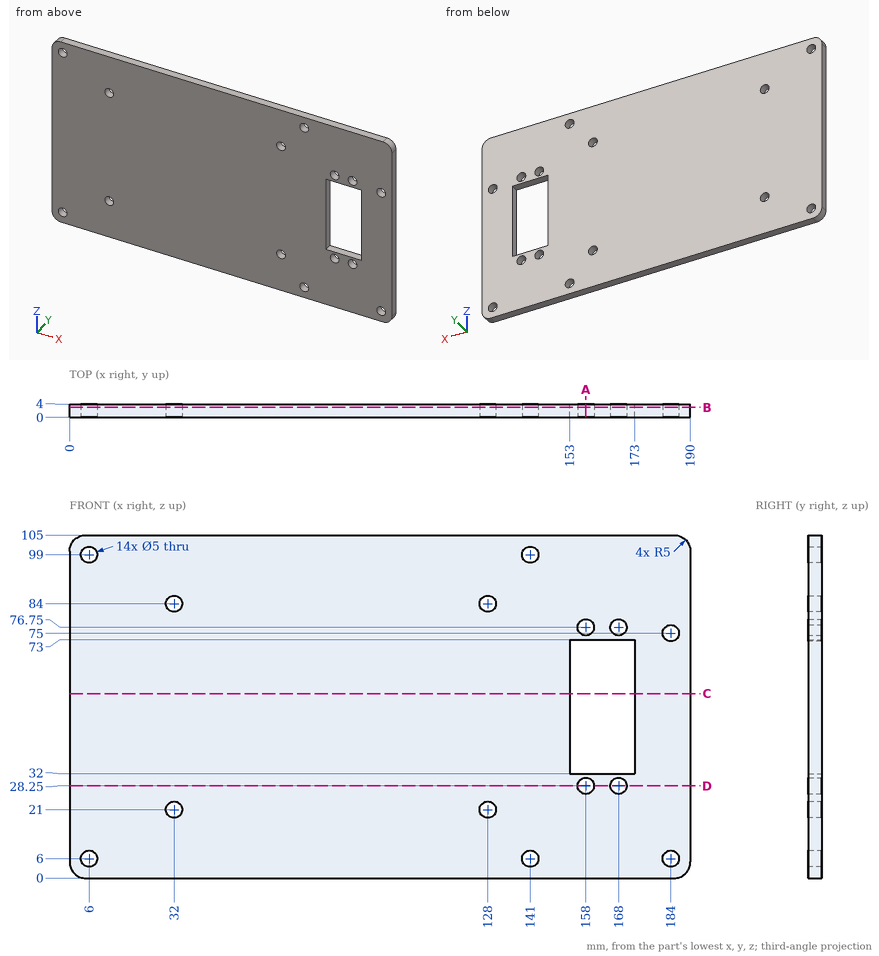
Design review of the part shown in the three views and the two pictorial views. Dimensions are in mm from the part's minimum x, y and z. Round coordinates to 2 decimals unless told otherwise and drop trailing zeros. Loops run counter-clockwise (first coordinate to the right, second up) from the corner with the lowest first, then second, coordinate; pieces in that order, holes last.
1) Wall thickness on line 1 along Z through (x, y) = (128, 3); line 2 along X through (y, z) = (2.55, 6); line 3 along X through (y, z) = (1.8, 84): over which ranges is each line inside the solid? List them lowest first.
Values follow:
line 1: z = 0 to 18.5, 23.5 to 81.5, 86.5 to 105
line 2: x = 0 to 3.5, 8.5 to 138.5, 143.5 to 181.5, 186.5 to 190
line 3: x = 0 to 29.5, 34.5 to 125.5, 130.5 to 190
2) Consider section D-D on z = 28.25. State the section outline as (x, y) points.
Values follow:
outline: (0, 0) - (155.5, 0) - (155.5, 4) - (0, 4) - close; (160.5, 0) - (165.5, 0) - (165.5, 4) - (160.5, 4) - close; (170.5, 0) - (190, 0) - (190, 4) - (170.5, 4) - close
3) Consider section B-B on y = 3. Give the number of separate pieces and of enclosed holes in the cut face, then the cut area to 3 significant figures.
Values follow:
separate pieces: 1
enclosed holes: 15
area: 18,800 mm2
4) Clearance check with a flat-ended pin moving along its axis: P1, Ø3, axis at x = 141, z = 6, coming from the -Y side. State where the tip first meets the part, or that it passes through.
Values follow:
P1: passes through
5) Consider section A-A on x = 158. State the section outline as (y, z) points, then the cut area to 3 significant figures.
Values follow:
outline: (0, 0) - (4, 0) - (4, 25.75) - (0, 25.75) - close; (0, 30.75) - (4, 30.75) - (4, 32) - (0, 32) - close; (0, 73) - (4, 73) - (4, 74.25) - (0, 74.25) - close; (0, 79.25) - (4, 79.25) - (4, 105) - (0, 105) - close
area: 216 mm2
6) Consider section C-C on z = 56.5. State the section outline as (x, y) points.
Values follow:
outline: (0, 0) - (153, 0) - (153, 4) - (0, 4) - close; (173, 0) - (190, 0) - (190, 4) - (173, 4) - close
